Source: CAD feature listing. Evaluate the final solid. Frame: model axes, mm. Round coordinates to 2 decimals unless told otherwise and drop trailing zeros. Loops run counter-clockwise (first coordinate to the right, second up) from the corner with the lowest first, then second, coordinate; pieces in that order, holes last. Notation, with made-up numbers: M -19,4.25 L 19,4.25 A14 ccw 19,26.25 Z; hole C 64.5,36.25 d5. An arc over 180 degrees is marked long. Write each question's results on one line, items separated by ' | '. Start each with the question number.
1. Section A-A on y = -1.6. Give the number of separate pieces and of enclosed holes in the cut face, and give its area (3 significant figures).
2. Section C-C on z = -105.5. Output: boundary loops of the cut face in (x, y) (3 decimals), and give its area (3 significant figures).
3. Section B-B on x = 37. Output: boundary loops of the cut face in (y, z) (3 decimals).
4. Ray query, line 1 (Z direction, x = 45, y = -0.7); line 2 (Z direction, x = 45.5, y = -2.9); line 3 (Z direction, x = 2, y = -1.75). Return the intervals inside material, ascending.
5. Contact query for a flat-ended pin moving along its axis: pin 1 Ø10 at (x, z) = (44.45, 0) entering from +Y. Output: stop coordinate, or through.
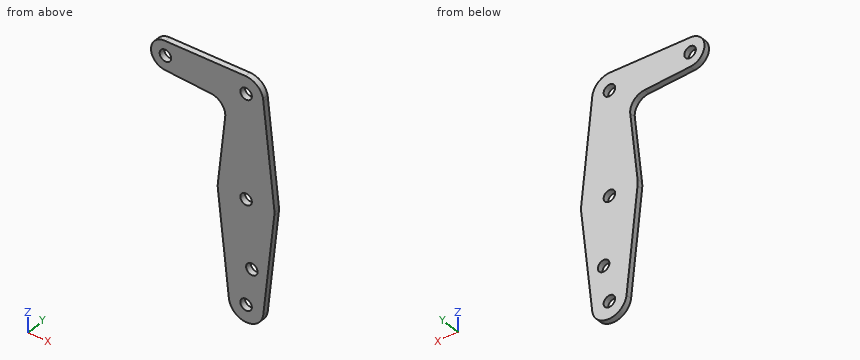
from build123d import *

# Parameters (mm, degrees)
F0_R     = 3.175
F1_DEPTH = 3.175


with BuildPart() as f1:
    # F0 (on Front) → F1 (new body)
    with BuildSketch(Plane.XZ):
        with BuildLine():
            ThreePointArc((0, -7.9375), (5.61266, -5.61266), (7.9375, 0))
            ThreePointArc((7.9375, 0), (5.61266, 5.61266), (0, 7.9375))
            ThreePointArc((0, 7.9375), (-7.9375, 0), (0, -7.9375))
        make_face()
        Circle(F0_R, mode=Mode.SUBTRACT)
        with BuildLine():
            ThreePointArc((59.980986, -55.475453), (44.445822, -41.529001), (28.91812, -55.48376))
            ThreePointArc((28.91812, -55.48376), (28.829, -57.15), (28.91812, -58.81624))
            ThreePointArc((28.91812, -58.81624), (44.45, -72.771), (59.98188, -58.81624))
            ThreePointArc((59.98188, -58.81624), (60.048704, -57.984311), (60.071, -57.15))
            ThreePointArc((60.071, -57.15), (60.04848, -56.311518), (59.980986, -55.475453))
        make_face()
        with Locations((44.45, -57.15)):
            Circle(F0_R, mode=Mode.SUBTRACT)
        with BuildLine():
            ThreePointArc((53.808394, 1.773721), (50.393401, 7.443226), (44.108729, 9.518884))
            ThreePointArc((44.108729, 9.518884), (37.836566, -6.854788), (53.975, 0))
            ThreePointArc((53.975, 0), (53.9741, 0.130959), (53.971399, 0.261894))
            Line((53.971399, 0.261894), (53.808394, 1.773721))
        make_face()
        with Locations((44.45, 0)):
            Circle(F0_R, mode=Mode.SUBTRACT)
        with BuildLine():
            ThreePointArc((53.975, -114.3), (43.941274, -104.788595), (34.979342, -115.316))
            ThreePointArc((34.979342, -115.316), (44.45, -123.825), (53.920658, -115.316))
            ThreePointArc((53.920658, -115.316), (53.961405, -114.808726), (53.975, -114.3))
        make_face()
        with Locations((44.45, -114.3)):
            Circle(F0_R, mode=Mode.SUBTRACT)
        with BuildLine():
            ThreePointArc((59.98188, -58.81624), (44.45, -72.771), (28.91812, -58.81624))
            Line((28.91812, -58.81624), (34.979342, -115.316))
            ThreePointArc((34.979342, -115.316), (43.941274, -104.788595), (53.975, -114.3))
            ThreePointArc((53.975, -114.3), (53.961405, -114.808726), (53.920658, -115.316))
            Line((53.920658, -115.316), (59.98188, -58.81624))
        make_face()
        with Locations((47.625, -93.6625)):
            Circle(F0_R, mode=Mode.SUBTRACT)
        with BuildLine():
            ThreePointArc((0, 7.9375), (5.61266, 5.61266), (7.9375, 0))
            ThreePointArc((7.9375, 0), (5.61266, -5.61266), (0, -7.9375))
            Line((0, -7.9375), (25.099068, -8.837351))
            ThreePointArc((25.099068, -8.837351), (30.996049, -11.659012), (32.950342, -17.897351))
            Line((32.950342, -17.897351), (28.91812, -55.48376))
            ThreePointArc((28.91812, -55.48376), (44.445822, -41.529001), (59.980986, -55.475453))
            Line((59.980986, -55.475453), (53.971399, 0.261894))
            ThreePointArc((53.971399, 0.261894), (53.9741, 0.130959), (53.975, 0))
            ThreePointArc((53.975, 0), (37.836566, -6.854788), (44.108729, 9.518884))
            Line((44.108729, 9.518884), (0, 7.9375))
        make_face()
    extrude(amount=F1_DEPTH)


solid = f1.part
Taken from the geometry:
1) separate pieces: 1 | enclosed holes: 5 | area: 3,740 mm^2
2) outline: M 33.926,-3.175 L 54.974,-3.175 L 54.974,0 L 33.926,0 Z | area: 66.8 mm^2
3) outline: M -3.175,-120.235 L 0,-120.235 L 0,9.264 L -3.175,9.264 Z
4) line 1: -123.81 to -117.43, -111.17 to -95.45, -91.88 to -60.28, -54.02 to -3.13, 3.13 to 9.51 | line 2: -123.77 to -117.3, -111.3 to -96.02, -91.3 to -60.15, -54.15 to -3, 3 to 9.47 | line 3: -8.01 to -2.47, 2.47 to 8.01
5) pin 1: y = 0
